Could you check a few things on this model? Use its own coordinates, in mm. A direction names the side the tool comes from. Coordinates: 2 decimals unless noted, no trailing zeros. Loops run counter-clockwise (first coordinate to the right, second up) from the corner with the lowest first, then second, coordinate; pieces in that order, holes last.
1) Imagine slicing it at D-D on y = 19. Please give me the cut outline in (x, z) (3 decimals), plus the area to 3 significant figures.
2) Thinking about a two-plate mould opening in Y: for faces 4 (the face through (-0.551, -46.733, 2.504)), 5 (the face through (0, 39.688, 13)), 6 (the face through (4.064, 43, 4)), which applies, released by +Y, released by -Y, zero draft, split by the parting line, or undercut?
3) Imagine slicing it at B-B on x = 0. Give the number of separate pieces and of enclosed holes in the cut face, plus the area to 3 significant figures.
4) Imagine slicing it at A-A on z = 3. Please give me the cut outline in (x, y), plus the area to 3 significant figures.
5) If I drill on line 1 along Y through (x, z) = (0, 3.7); line 2 along Y through (x, z) = (2.75, 12.25); line 3 along Y through (x, z) = (1.75, 2.25), over which ranges is the centre line in solid material (lowest first)?
6) Will these pins go through, and if not, where does the flat tip stop? P1, Ø3, axis at x = 0, y = 49.21, coming from the +Z side; P2, Ø4, axis at x = 1.5, z = 10.5, coming from the -Y side; P3, Ø0.9, axis at x = 0.5, z = 13.5, coming from the -Y side; P4, Ø2, axis at x = 1.5, z = 10, coming from the +Y side.
7) Imagine slicing it at C-C on y = -41. Please give me the cut outline in (x, z), plus the area to 3 significant figures.
8) For faces 1 (the face through (1.71, -0.51, 12.2)), 2 (the face through (0, -39.688, 13)), 3 (the face through (-0.331, 46.694, 2.504)), which set-ups out of +Z, -Z, +X, -X, +Y, -Y let a thin tool reach every point of the face, with its end or its side?
```python
from build123d import *

# Parameters (mm, degrees)
F0_R     = 3.175
F1_DEPTH = 39.6875
F2_W     = 73.025
F2_H     = 18.185855
F3_DEPTH = 12.7
F4_R     = 3.175
F5_DEPTH = 79.375
F6_W     = 9.525
F6_H     = 3.175
F7_DEPTH = 12.7
F8_R     = 2.54
F9_DEPTH = 6.35
F10_R    = 5.08
F11_SIZE = 1.27


with BuildPart() as f1:
    # F0 (on Front) → F1 (new body, symmetric)
    with BuildSketch(Plane.XZ):
        with BuildLine():
            Line((4.064, 0), (4.064, 10.414))
            ThreePointArc((4.064, 10.414), (0, 14.478), (-4.064, 10.414))
            Line((-4.064, 10.414), (-4.064, 0))
            Line((-4.064, 0), (4.064, 0))
        make_face()
        with Locations((0, 9.525)):
            Circle(F0_R, mode=Mode.SUBTRACT)
    extrude(amount=F1_DEPTH, both=True)

    # F2 (on Right) → F3 (cut, symmetric)
    with BuildSketch(Plane.YZ):
        with Locations((0, 6.139678)):
            Rectangle(F2_W, F2_H)
    extrude(amount=F3_DEPTH, both=True, mode=Mode.SUBTRACT)

    # F4 (on face) → F5 (join)
    with BuildSketch(Plane.XZ.offset(39.6875)):
        with Locations((0, 9.525)):
            Circle(F4_R)
    extrude(amount=-F5_DEPTH)

    # F6 (on Right) → F7 (cut, symmetric)
    with BuildSketch(Plane.YZ):
        with Locations((-30.7975, 2.8575)):
            Rectangle(F6_W, F6_H)
        with Locations((30.7975, 2.8575)):
            Rectangle(F6_W, F6_H)
    extrude(amount=F7_DEPTH, both=True, mode=Mode.SUBTRACT)

    # F8 (on face) → F9 (join)
    with BuildSketch(Plane(origin=(0, 0, 0), x_dir=(1, 0, 0), z_dir=(0, 0, -1))):
        with BuildLine():
            Line((-4.064, 36.5125), (4.064, 36.5125))
            Line((4.064, 36.5125), (4.064, 49.2125))
            ThreePointArc((4.064, 49.2125), (0, 53.2765), (-4.064, 49.2125))
            Line((-4.064, 49.2125), (-4.064, 36.5125))
        make_face()
        with Locations((0, 49.2125)):
            Circle(F8_R, mode=Mode.SUBTRACT)
        with BuildLine():
            ThreePointArc((-4.064, -49.2125), (0, -53.2765), (4.064, -49.2125))
            Line((4.064, -49.2125), (4.064, -36.5125))
            Line((4.064, -36.5125), (-4.064, -36.5125))
            Line((-4.064, -36.5125), (-4.064, -49.2125))
        make_face()
        with Locations((0, -49.2125)):
            Circle(F8_R, mode=Mode.SUBTRACT)
    extrude(amount=-F9_DEPTH)

    # F10
    f10_edges = [f1.edges().sort_by_distance(p)[0] for p in [
        (0, 39.6875, 6.35),
        (0, -39.6875, 6.35),
    ]]
    fillet(f10_edges, radius=F10_R)

    # F11
    f11_edges = [f1.edges().sort_by_distance(p)[0] for p in [
        (-2.54, -49.2125, 6.35),
        (-2.54, 49.2125, 6.35),
    ]]
    chamfer(f11_edges, length=F11_SIZE)


solid = f1.part
```
Filled in:
1. outline: circle Ø6.35 at (0, 9.525)
1. area: 31.7 mm2
2. face 4: undercut
2. face 5: released by +Y
2. face 6: zero draft
3. separate pieces: 3
3. enclosed holes: 0
3. area: 672 mm2
4. outline: (-4.06, -49.21) arc R4.06 ccw to (4.06, -49.21) - (4.06, -36.51) - (-4.06, -36.51) - close; (-4.06, 36.51) - (4.06, 36.51) - (4.06, 49.21) arc R4.06 ccw to (-4.06, 49.21) - close; hole circle Ø5.08 at (0, -49.21); hole circle Ø5.08 at (0, 49.21)
4. area: 218 mm2
5. line 1: y = -53.28 to -51.75, -46.67 to -36.51, 36.51 to 46.67, 51.75 to 53.28
5. line 2: y = -39.69 to -36.51, 36.51 to 39.69
5. line 3: y = -52.88 to -51.05, -47.37 to -36.51, 36.51 to 47.37, 51.05 to 52.88
6. P1: passes through
6. P2: stops at y = -40.62
6. P3: stops at y = -39.69
6. P4: stops at y = 40.31
7. outline: (-4.06, 0) - (4.06, 0) - (4.06, 8.02) - (-4.06, 8.02) - close
7. area: 65.2 mm2
8. face 1: none
8. face 2: +Z, +X, -X, -Y
8. face 3: +Z, -Z
